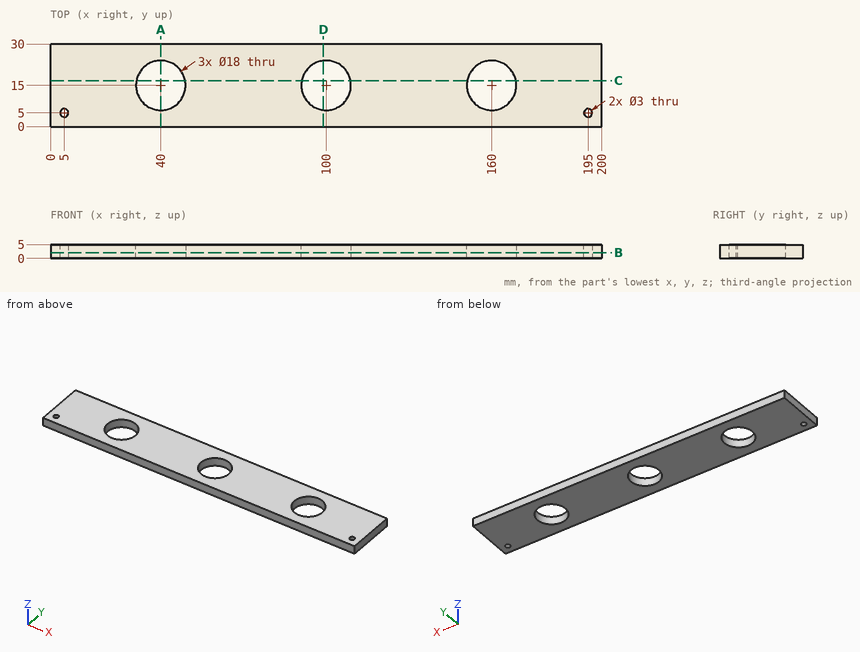
Source: three-view drawing plus pictorial views. Frame: mm from the lowest corner of the part. Coordinates: 2 decimals unless noted, no trailing zeros. Order: outer loops, then holes, each group sorted by start corner. A loop starts at its lowest first (then second) coordinate and runs counter-clockwise, first axis right, second up.
Item 1: Cut plane D-D (x = 99). Return loops of the section in (y, z).
Output values:
outline: (0, 0) - (6.06, 0) - (6.06, 5) - (0, 5) - close; (23.94, 0) - (30, 0) - (30, 5) - (23.94, 5) - close
Item 2: Cut plane A-A (x = 40). Return loops of the section in (y, z), plus the area to 3 significant figures.
Output values:
outline: (0, 0) - (6, 0) - (6, 5) - (0, 5) - close; (24, 0) - (30, 0) - (30, 5) - (24, 5) - close
area: 60.0 mm2
Item 3: Cut plane B-B (z = 2.15). Return loops of the section in (x, y).
Output values:
outline: (0, 0) - (200, 0) - (200, 30) - (0, 30) - close; hole circle Ø3 at (5, 5); hole circle Ø18 at (40, 15); hole circle Ø18 at (100, 15); hole circle Ø18 at (160, 15); hole circle Ø3 at (195, 5)
Item 4: First-contact query: P1, Ø11, axis at x = 100, y = 15, coming from the -Z side. Flat tip, straight axial feed; report the tip coordinate or a pass-through.
Output values:
P1: passes through
Item 5: Cut plane C-C (y = 16.75). Return loops of the section in (x, z).
Output values:
outline: (0, 0) - (31.17, 0) - (31.17, 5) - (0, 5) - close; (48.83, 0) - (91.17, 0) - (91.17, 5) - (48.83, 5) - close; (108.83, 0) - (151.17, 0) - (151.17, 5) - (108.83, 5) - close; (168.83, 0) - (200, 0) - (200, 5) - (168.83, 5) - close
Item 6: Material intervals for line 1 (X direction, y = 5.25, z = 3.15); line 2 (X direction, y = 9.5, z = 3.35); line 3 (X direction, y = 12.5, z = 1.15), sorted ascending.
Output values:
line 1: x = 0 to 3.52, 6.48 to 193.52, 196.48 to 200
line 2: x = 0 to 32.88, 47.12 to 92.88, 107.12 to 152.88, 167.12 to 200
line 3: x = 0 to 31.35, 48.65 to 91.35, 108.65 to 151.35, 168.65 to 200
